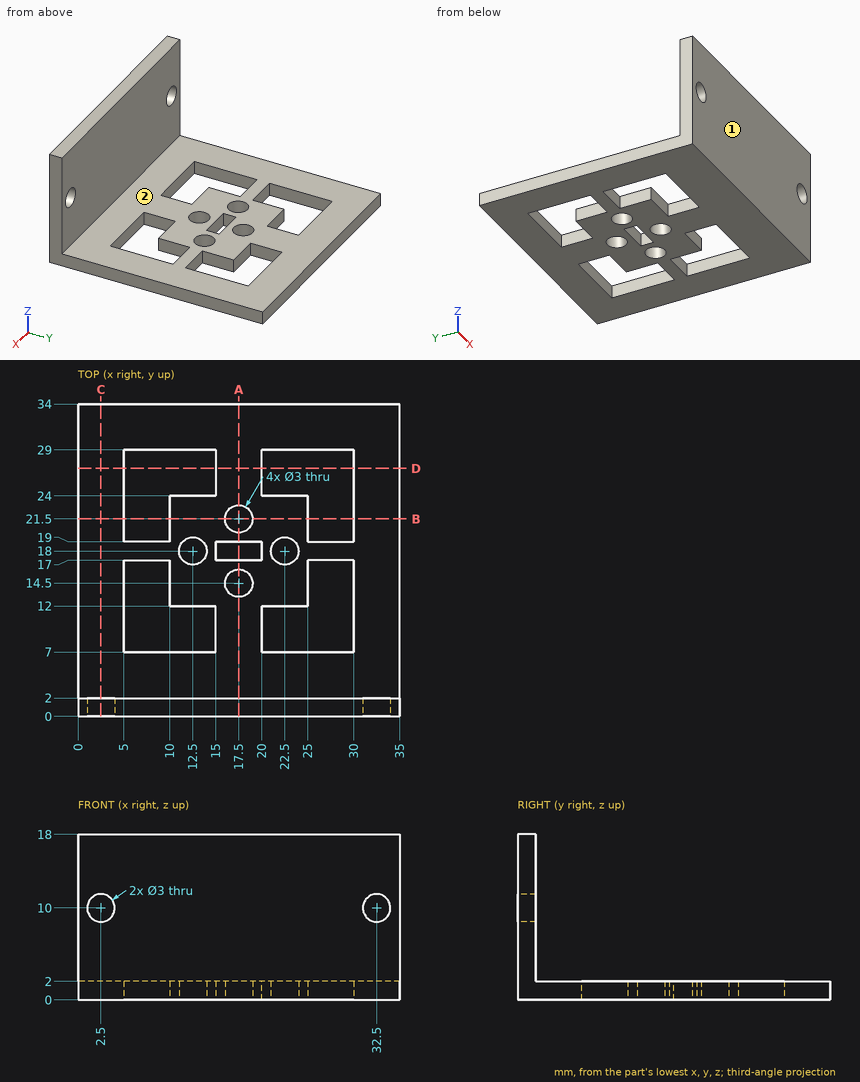
Source: three-view drawing plus pictorial views. Frame: mm from the lowest corner of the part. A direction names the side the tool comes from. Give positions to 0.01 mm unless a question says otherwise; leave off trailing zeros. Loops run counter-clockwise (first coordinate to the right, second up) from the corner with the lowest first, then second, coordinate; pieces in that order, holes last. Notation, with made-up numbers: (-34, 25) -> (-4, 25) arc R16 cw to (-4, 32) -> close; hole circle Ø11 at (79, 70.25). An arc over 180 degrees is marked (long way). Use a Markdown table: item, result. Add a question column.
(1) Section query C-C (x = 2.5). Output: boundary loops of the cut face in (y, z), then the cut area to 3 significant figures.
(2) Section query A-A (x = 17.5). Output: boundary loops of the cut face in (y, z), then the cut area to 3 significant figures.
(3) First-contact query: pin 1 Ø10 at (y, z) = (22, 11.5) entering from -X; pin 2 Ø10 at (x, z) = (5.5, 7.5) entering from +Y; pin 3 Ø5 at (x, y) = (25, 19) entering from +Z. Flat tips, straight axial feed; report the tip coordinate or a pass-through.
(4) Ray query, line 1 (Y direction, x = 24.5, z = 1.5); line 2 (Y direction, x = 12.5, z = 0.8); line 3 (X direction, y = 1.55, z = 10). Return the intervals inside material, ascending.
(5) Section query B-B (y = 21.5). Output: boundary loops of the cut face in (x, z), then the cut area to 3 significant figures.
(6) Section query D-D (y = 27). Output: boundary loops of the cut face in (x, z), then the cut area to 3 significant figures.
(7) Access query for the marked faces 1 and 2. Directions: +Z, -Z, +X, -X, +Y, -Y. A direction counts if a zero-diameter tool reaches every point of the face in a straight line with its end or side. Return the directions, or none.
Checked values:
| question | item | result |
|---|---|---|
| 1 | outline | (0, 0) -> (34, 0) -> (34, 2) -> (2, 2) -> (2, 8.5) -> (0, 8.5) -> close; (0, 11.5) -> (2, 11.5) -> (2, 18) -> (0, 18) -> close |
| 1 | area | 94.0 mm^2 |
| 2 | outline | (0, 0) -> (13, 0) -> (13, 2) -> (2, 2) -> (2, 18) -> (0, 18) -> close; (16, 0) -> (17, 0) -> (17, 2) -> (16, 2) -> close; (19, 0) -> (20, 0) -> (20, 2) -> (19, 2) -> close; (23, 0) -> (34, 0) -> (34, 2) -> (23, 2) -> close |
| 2 | area | 84.0 mm^2 |
| 3 | pin 1 | through |
| 3 | pin 2 | y = 2 |
| 3 | pin 3 | z = 2 |
| 4 | line 1 | 0 to 7, 12 to 24, 29 to 34 |
| 4 | line 2 | 0 to 7, 12 to 16.5, 19.5 to 24, 29 to 34 |
| 4 | line 3 | 0 to 1, 4 to 31, 34 to 35 |
| 5 | outline | (0, 0) -> (5, 0) -> (5, 2) -> (0, 2) -> close; (10, 0) -> (16, 0) -> (16, 2) -> (10, 2) -> close; (19, 0) -> (25, 0) -> (25, 2) -> (19, 2) -> close; (30, 0) -> (35, 0) -> (35, 2) -> (30, 2) -> close |
| 5 | area | 44.0 mm^2 |
| 6 | outline | (0, 0) -> (5, 0) -> (5, 2) -> (0, 2) -> close; (15, 0) -> (20, 0) -> (20, 2) -> (15, 2) -> close; (30, 0) -> (35, 0) -> (35, 2) -> (30, 2) -> close |
| 6 | area | 30.0 mm^2 |
| 7 | face 1 | +Z, -Z, +X, -X, -Y |
| 7 | face 2 | +Z, +X, -X, +Y |
